Could you check a few things on this model? Use its own coordinates, in mm. A direction names the side the tool comes from. Round coordinates to 2 decimals unless told otherwise and drop trailing zeros. Write each loop counter-clockwise with the first axis right and the second up, starting at its lowest first coordinate (ties: lowest second). Pieces come first, ordered by that corner, then holes.
```python
from build123d import *

# Parameters (mm, degrees)
SKETCH1_W           = 30.48
SKETCH1_H           = 17.78
BOSS_EXTRUDE1_DEPTH = 5.08
SKETCH3_R           = 1.5875
CUT_EXTRUDE1_DEPTH  = 36.101886702
BOSS_EXTRUDE2_START = 5.08
SKETCH4_R           = 2.496623085
SKETCH4_R_2         = 1.5875
SKETCH4_R_3         = 2.54
BOSS_EXTRUDE2_DEPTH = 5.08
SKETCH6_W           = 26.095055506
SKETCH6_H           = 8.553777079
SKETCH6_R           = 1.646398399
BOSS_EXTRUDE3_DEPTH = 5.08
SKETCH7_W           = 57.960584247
SKETCH7_H           = 6.84758287
SKETCH7_R           = 1.709119501
BOSS_EXTRUDE4_DEPTH = 5.08


with BuildPart() as part:
    # Sketch1 → Boss-Extrude1 (new body)
    with BuildSketch(Plane(origin=(0, 0, 0), x_dir=(1, 0, 0), z_dir=(0, 1, 0))):
        with Locations((14.675357499, -8.756740088)):
            Rectangle(SKETCH1_W, SKETCH1_H)
    extrude(amount=BOSS_EXTRUDE1_DEPTH)

    # Sketch3 → Cut-Extrude1 (cut, through all)
    with BuildSketch(Plane(origin=(0, 5.08, 0), x_dir=(1, 0, 0), z_dir=(0, 1, 0))):
        with Locations(Location((1.975357499, -2.406740088, 0), (0, 0, 270))):
            Circle(SKETCH3_R)
        with Locations(Location((27.375357499, -15.106740088, 0), (0, 0, 270))):
            Circle(SKETCH3_R)
    extrude(amount=-CUT_EXTRUDE1_DEPTH, mode=Mode.SUBTRACT)

    # Sketch4 → Boss-Extrude2 (add)
    # profile 1 of 2: a face of its own
    with BuildSketch(Plane(origin=(0, 5.08, 0), x_dir=(1, 0, 0), z_dir=(0, 1, 0)).offset(BOSS_EXTRUDE2_START)):
        with Locations(Location((1.975357499, -2.406740088, 0), (0, 0, 270))):
            Circle(SKETCH4_R)
        with Locations(Location((1.975357499, -2.406740088, 0), (0, 0, 270))):
            Circle(SKETCH4_R_2, mode=Mode.SUBTRACT)
    # profile 2 of 2: a face of its own
    with BuildSketch(Plane(origin=(0, 5.08, 0), x_dir=(1, 0, 0), z_dir=(0, 1, 0)).offset(BOSS_EXTRUDE2_START)):
        with Locations(Location((27.375357499, -15.106740088, 0), (0, 0, 270))):
            Circle(SKETCH4_R_3)
        with Locations(Location((27.375357499, -15.106740088, 0), (0, 0, 270))):
            Circle(SKETCH4_R_2, mode=Mode.SUBTRACT)
    extrude(amount=-BOSS_EXTRUDE2_DEPTH)

    # Sketch6 → Boss-Extrude3 (add)
    with BuildSketch(Plane(origin=(0, 5.08, 0), x_dir=(1, 0, 0), z_dir=(0, 1, 0))):
        with Locations((42.962885252, -5.938189685)):
            Rectangle(SKETCH6_W, SKETCH6_H)
        with Locations(Location((50.930413005, -6.484145564, 0), (0, 0, 270))):
            Circle(SKETCH6_R, mode=Mode.SUBTRACT)
    extrude(amount=-BOSS_EXTRUDE3_DEPTH)

    # Sketch7 → Boss-Extrude4 (add)
    with BuildSketch(Plane(origin=(0, 5.08, 0), x_dir=(1, 0, 0), z_dir=(0, 1, 0))):
        with Locations((-29.309294872, -6.791286789)):
            Rectangle(SKETCH7_W, SKETCH7_H)
        with Locations(Location((-53.209586995, -6.405078224, 0), (0, 0, 270))):
            Circle(SKETCH7_R, mode=Mode.SUBTRACT)
    extrude(amount=-BOSS_EXTRUDE4_DEPTH)


solid = part.part
```
Q1. Imagine slicing it at A-A, the plane z = 6. Write out the boundary of the cut face in (x, y).
Q2. Imagine slicing it at B-B, the plane y = 7.5. Write out the boundary of the cut face in (x, z) (1 decimal), then the cut area to 3 significant figures.
Q3. On a 3-axis mill with a long thin cutter (end or side, diameter ignored), from which of +Z, -Z, +X, -X, +Y, -Y can I reach the whole of each face in a straight line? I mean faces 1 (the flat face through (29.4, 5.08, 17.1)), 2 (the flat face through (43, 3, 1.661)), 3 (the flat face through (-30, 3, 3.367)), 4 (the flat face through (-0.565, 3, 14)), 5 (the cylindrical face through (0.456, 7.656, 0.426)). Say none if no direction works.
Q4. We'd pull the mould along X, two halves only. Please class faces 6 (the cylindrical face through (28.45, 5.15, 13.94)), 7 (the flat face through (56.01, 3, 6)), 8 (the cylindrical face through (29.5, 7.7, 16.5)), 9 (the flat face through (43, 3, 10.215)): pulls with the +X half, pulls with the -X half, needs draft (parallel to the pull), parting line crosses it, or undercut.
Q5. I'm going to push flat-ended pins straight in: pin 1 Ø5 at (x, z) = (19, 3) entering from +Y; pin 2 Ø2.5 at (y, z) = (2, 13.5) entering from +X; pin 3 Ø2 at (y, z) = (8.5, 3) entering from -X. Where does each tip first touch, or does it pass through?
Q6. Imagine slicing it at D-D, the plane z = 11.5. Write out the boundary of the cut face in (x, y).
Q7. Imagine slicing it at C-C, the plane x = -14.5. Write out the boundary of the cut face in (y, z), then the cut area to 3 significant figures.
Q8. If I drill on L1, parallel to X at y = 2, z = 15.25; L2, parallel to X at y = 4.25, z = 5.5; L3, parallel to X at y = 1, z = 7, over which ranges is the centre line in solid material (lowest first)?
Results found:
1. outline: (-58.29, 0) - (-54.87, 0) - (-54.87, 5.08) - (-58.29, 5.08) - close; (-51.55, 0) - (49.36, 0) - (49.36, 5.08) - (-51.55, 5.08) - close; (52.5, 0) - (56.01, 0) - (56.01, 5.08) - (52.5, 5.08) - close
2. outline: circle Ø5 at (2, 2.4); circle Ø5.1 at (27.4, 15.1); hole circle Ø3.2 at (2, 2.4); hole circle Ø3.2 at (27.4, 15.1)
2. area: 24.0 mm2
3. face 1: +Z, +X, +Y
3. face 2: -Z, +X, +Y, -Y
3. face 3: -Z, -X, +Y, -Y
3. face 4: +Z, -X, +Y, -Y
3. face 5: +Y
4. face 6: undercut
4. face 7: pulls with the +X half
4. face 8: parting line crosses it
4. face 9: needs draft
5. pin 1: stops at y = 5.08
5. pin 2: stops at x = 29.92
5. pin 3: stops at x = -0.52
6. outline: (-0.56, 0) - (29.92, 0) - (29.92, 5.08) - (-0.56, 5.08) - close
7. outline: (0, 3.37) - (5.08, 3.37) - (5.08, 10.22) - (0, 10.22) - close
7. area: 34.8 mm2
8. L1: x = -0.56 to 25.79, 28.96 to 29.92
8. L2: x = -58.29 to -54.66, -51.76 to 49.61, 52.25 to 56.01
8. L3: x = -58.29 to -54.81, -51.61 to 49.37, 52.49 to 56.01
